from build123d import *

# Parameters (mm, degrees)
SKETCH1_R                                = 17.5
BOSS_EXTRUDE1_DEPTH                      = 5
CBORE_FOR_M3_PAN_HEAD_SCREW1_D           = 3.4
CBORE_FOR_M3_PAN_HEAD_SCREW1_CBORE_D     = 7
CBORE_FOR_M3_PAN_HEAD_SCREW1_CBORE_DEPTH = 2.4
CIRPATTERN1_COUNT                        = 3
F_12_0_12_DIAMETER_HOLE1_D               = 12
CUT_EXTRUDE1_DEPTH                       = 1.5
CIRPATTERN2_COUNT                        = 6


with BuildPart() as part:
    # Sketch1 → Boss-Extrude1 (new body)
    with BuildSketch(Plane(origin=(0, 0, 0), x_dir=(1, 0, 0), z_dir=(0, 1, 0))):
        with Locations(Location((0, 0, 0), (0, 0, 270))):
            Circle(SKETCH1_R)
    extrude(amount=BOSS_EXTRUDE1_DEPTH)

    # CBORE for M3 Pan Head Screw1 (through all)
    with Locations(Plane(origin=(0, 5, 0), x_dir=(1, 0, 0), z_dir=(0, 1, 0))):
        with Locations((-12, 0)):
            cbore_for_m3_pan_head_screw1 = CounterBoreHole(CBORE_FOR_M3_PAN_HEAD_SCREW1_D / 2, CBORE_FOR_M3_PAN_HEAD_SCREW1_CBORE_D / 2, CBORE_FOR_M3_PAN_HEAD_SCREW1_CBORE_DEPTH)

    # CirPattern1: CBORE for M3 Pan Head Screw1 ×3 about axis
    cirpattern1_axis = Axis((0, 0, 0), (0, 1, 0))
    for i in range(1, CIRPATTERN1_COUNT):
        add(cbore_for_m3_pan_head_screw1.rotate(cirpattern1_axis, i * 360 / CIRPATTERN1_COUNT), mode=Mode.SUBTRACT)

    # Ø12.0 (12) Diameter Hole1 (through all)
    with Locations(Plane(origin=(0, 0, 0), x_dir=(-1, 0, 0), z_dir=(0, -1, 0))):
        with Locations((0, 0)):
            Hole(F_12_0_12_DIAMETER_HOLE1_D / 2)

    # Sketch7 → Cut-Extrude1 (cut)
    with BuildSketch(Plane.XZ):
        Polygon((0, 25), (-5.723634799, 1.800001303), (5.723634799, 1.800001303), align=None)
    cut_extrude1 = extrude(amount=-CUT_EXTRUDE1_DEPTH, mode=Mode.SUBTRACT)

    # CirPattern2: Cut-Extrude1 ×6 about axis
    cirpattern2_axis = Axis((0, 0, 0), (0, 1, 0))
    for i in range(1, CIRPATTERN2_COUNT):
        add(cut_extrude1.rotate(cirpattern2_axis, i * 360 / CIRPATTERN2_COUNT), mode=Mode.SUBTRACT)


solid = part.part
Input: part model. Units: mm. Frame: model coordinates. A direction names the side the tool comes from. Coordinates: 2 decimals unless noted, no trailing zeros. Loops run counter-clockwise (first coordinate to the right, second up) from the corner with the lowest first, then second, coordinate; pieces in that order, holes last. Notation, with made-up numbers: (62, -32) -> (115, -32) arc R31 cw to (115, 6) -> close; hole circle Ø5 at (55, -26.75). An arc over 180 degrees is marked (long way). Write each question's results on one line, items separated by ' | '. Start each with the question number.
Q1. Reachability of faces 3 (the flat face through (-9.157, 0.74, 8.884)), 4 (the flat face through (-10, 2.6, -1)), 5 (the flat face through (4, 1.5, -6)), 6 (the cylindrical face through (6.369, 1.282, -8.733)) from +Z, -Z, +X, -X, +Y, -Y: full face, straight path, thin tool, end or side. Return the list, or none.
Q2. Section D-D, the plane z = 12.5. Return the cut outline in (x, y), plus the area to 3 significant figures.
Q3. Section B-B, the plane z = -4. Return the cut outline in (x, y), plus the area to 3 significant figures.
Q4. Pull-direction query (Z, two-part tool) for faces 1 (the flat face through (3.115, 0.74, 12.372)), 2 (the flat face through (7, 0, 12)); classes: released by +Z, released by -Z, zero draft, split by the parting line, or undercut.
Q5. Section C-C, the plane y = 3.25. Return the cut outline in (x, z).
Q6. Pin query (flat end, axial travel): pin 1 (1 mm diameter, centred on y = 1, z = -3, fed in from +X); pin 2 (5.5 mm diameter, centred on x = 6, z = -10.39, fed in from +Y); pin 3 (1 mm diameter, centred on x = -7.5, y = 0.5, fed in from +Z); pin 4 (6.5 mm diameter, centred on x = 6, z = -10.39, fed in from -Y). Return the tip coordinate at first contact, or that it passes through.
Q7. Ray query, line 1 (X direction, y = 3, z = -3); line 2 (Z direction, x = -12, y = 0.65); line 3 (Y direction, x = 5, z = -6.5). Return the intervals inside material, ascending. Write a range as from..to.
Q8. Section A-A, the plane x = 0. Return the cut outline in (y, z), plus the area to 3 significant figures.
Found:
1) face 3: -X, -Y | face 4: +Y | face 5: -Y | face 6: +Y, -Y
2) outline: (-12.25, 0) -> (-3.08, 0) -> (-3.08, 1.5) -> (3.08, 1.5) -> (3.08, 0) -> (12.25, 0) -> (12.25, 5) -> (8.79, 5) -> (8.79, 2.6) -> (3.21, 2.6) -> (3.21, 5) -> (-12.25, 5) -> close | area: 99.8 mm2
3) outline: (-17.04, 0) -> (-12.81, 0) -> (-12.81, 1.5) -> (-4.47, 1.5) -> (-4.47, 5) -> (-17.04, 5) -> close; (4.47, 1.5) -> (12.81, 1.5) -> (12.81, 0) -> (17.04, 0) -> (17.04, 5) -> (4.47, 5) -> close | area: 101 mm2
4) face 1: undercut | face 2: zero draft
5) outline: circle Ø35 at (0, 0); hole circle Ø7 at (-12, 0); hole circle Ø12 at (0, 0); hole circle Ø7 at (6, -10.39); hole circle Ø7 at (6, 10.39)
6) pin 1: x = 17.32 | pin 2: y = 2.6 | pin 3: z = 16.04 | pin 4: y = 0
7) line 1: -17.24..-13.8, -10.2..-5.2, 5.2..17.24 | line 2: -12.74..-9.71, -3.23..-1.7, 1.7..3.23, 9.71..12.74 | line 3: 1.5..5
8) outline: (1.5, -17.5) -> (5, -17.5) -> (5, -6) -> (1.5, -6) -> close; (1.5, 6) -> (5, 6) -> (5, 17.5) -> (1.5, 17.5) -> close | area: 80.5 mm2
